Verification items for the finished model (mm, model axes). Round coordinates to 2 decimals unless told otherwise and drop trailing zeros. Write each loop counter-clockwise with the first axis right and the second up, starting at its lowest first coordinate (ties: lowest second). Pieces come first, ordered by that corner, then holes. Notation, with made-up numbers: M -32,-15 L -7,-15 A25 cw -7,10 Z; hole C 69.5,54 d1. An arc over 180 degrees is marked long. One line per item, written item: value. Start each with the question number.
from build123d import *

# Parameters (mm, degrees)
F2_DEPTH = 4.7625
F1_R     = 6.35
F1_R_2   = 1.5875
F1_R_3   = 3.175
F1_R_4   = 5.55625
F1_R_5   = 5.159375
F1_R_6   = 4.7625
F1_R_7   = 4.365625
F1_R_8   = 3.96875
F1_R_9   = 3.571875
F1_R_10  = 2.778125
F1_R_11  = 2.38125
F1_R_12  = 1.984375
F3_DEPTH = 35.56


with BuildPart() as f2:
    # F0 (on Top) → F2 (new body)
    with BuildSketch(Plane.XY):
        with BuildLine():
            Line((83.220267, 40.4495), (-46.799858, 40.4495))
            ThreePointArc((-46.799858, 40.4495), (-70.588232, 15.0495), (-46.799858, -10.3505))
            Line((-46.799858, -10.3505), (83.220267, -10.3505))
            ThreePointArc((83.220267, -10.3505), (87.710395, -8.490628), (89.570267, -4.0005))
            Line((89.570267, -4.0005), (89.570267, 34.0995))
            ThreePointArc((89.570267, 34.0995), (87.710395, 38.589628), (83.220267, 40.4495))
        make_face()
    extrude(amount=F2_DEPTH)

    # F1 (on face) → F3 (cut)
    with BuildSketch(Plane.XY):
        with Locations((-24.940642, 27.7495)):
            Circle(F1_R)
        with Locations((-24.940642, 2.3495)):
            Circle(F1_R_2)
        with Locations((-48.657889, 15.0495)):
            Circle(F1_R_3)
        with Locations((-5.890642, 27.7495)):
            Circle(F1_R_4)
        with Locations((13.159358, 27.7495)):
            Circle(F1_R_5)
        with Locations((32.209358, 27.7495)):
            Circle(F1_R_6)
        with Locations((51.259358, 27.7495)):
            Circle(F1_R_7)
        with Locations((70.309358, 27.7495)):
            Circle(F1_R_8)
        with Locations((70.309358, 2.3495)):
            Circle(F1_R_9)
        with Locations((51.259358, 2.3495)):
            Circle(F1_R_3)
        with Locations((32.209358, 2.3495)):
            Circle(F1_R_10)
        with Locations((13.159358, 2.3495)):
            Circle(F1_R_11)
        with Locations((-5.890642, 2.3495)):
            Circle(F1_R_12)
    extrude(amount=F3_DEPTH, mode=Mode.SUBTRACT)


solid = f2.part
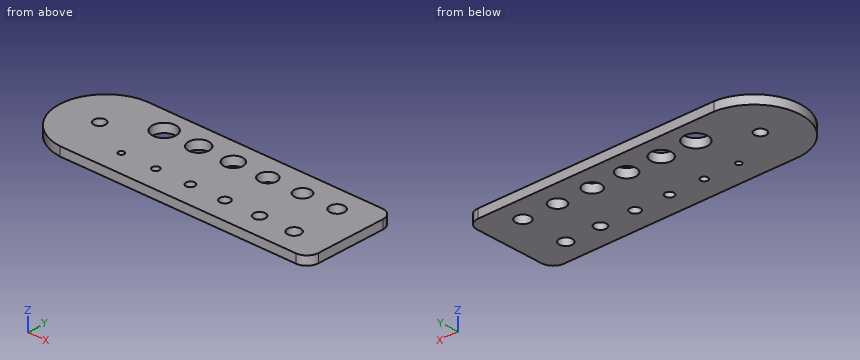
1) Cross-section at B-B (y = 30). Record the boundary of the cut face in (x, z).
2) Cross-section at A-A (x = 32). Record the boundary of the cut face in (y, z), then the cut area to 3 significant figures.
3) Cross-section at C-C (z = 2.45). State how many separate pieces and enclosed holes the cut face has, then the cut area to 3 significant figures.
4) Thickness scan on line 1 (Y direction, x = 31, z = 2.8); line 2 (Y direction, x = 30.5, z = 3.4); line 3 (X direction, y = 16.5, z = 1). Record the ranges inside material, lowest first.
5) Gauge pin test, flat end, axial feed: pin 1 Ø5 at (x, y) = (51.26, 2.35) entering from -Z. Record the tip position at first contact, or that the pin passes through.
6) Cross-section at D-D (x = -50). Record the boundary of the cut face in (y, z).
Results below:
1. outline: M -65.74,0 L -30.88,0 L -30.88,4.76 L -65.74,4.76 Z; M -19,0 L -10.97,0 L -10.97,4.76 L -19,4.76 Z; M -0.81,0 L 8.52,0 L 8.52,4.76 L -0.81,4.76 Z; M 17.8,0 L 28.01,0 L 28.01,4.76 L 17.8,4.76 Z; M 36.41,0 L 47.52,0 L 47.52,4.76 L 36.41,4.76 Z; M 55,0 L 67.04,0 L 67.04,4.76 L 55,4.76 Z; M 73.58,0 L 89.57,0 L 89.57,4.76 L 73.58,4.76 Z
2. outline: M -10.35,0 L -0.42,0 L -0.42,4.76 L -10.35,4.76 Z; M 5.12,0 L 22.99,0 L 22.99,4.76 L 5.12,4.76 Z; M 32.51,0 L 40.45,0 L 40.45,4.76 L 32.51,4.76 Z
2. area: 170 mm²
3. separate pieces: 1
3. enclosed holes: 13
3. area: 7,190 mm²
4. line 1: y = -10.35 to -0.15, 4.85 to 23.14, 32.36 to 40.45
4. line 2: y = -10.35 to 0.16, 4.54 to 23.3, 32.19 to 40.45
4. line 3: x = -70.55 to -51.48, -45.83 to 89.57
5. pin 1: passes through
6. outline: M -9.94,0 L 12.17,0 L 12.17,4.76 L -9.94,4.76 Z; M 17.93,0 L 40.03,0 L 40.03,4.76 L 17.93,4.76 Z
